Check sheet for the drawn part. Datum: minimum x, y, z corner. Units: mm. A direction names the side the tool comes from. Give positions to 0.01 mm unless a question says otherwise; leave off trailing zeros. Loops run counter-clockwise (first coordinate to the right, second up) from the corner with the lowest first, then second, coordinate; pieces in that order, holes last. Notation, with made-up numbers: (-40, 0.5) -> (7, 0.5) arc R21 ccw to (7, 16.5) -> close; hole circle Ø5 at (69, 83). An arc over 180 degrees is marked (long way). One line per question, with ' | ' between items.
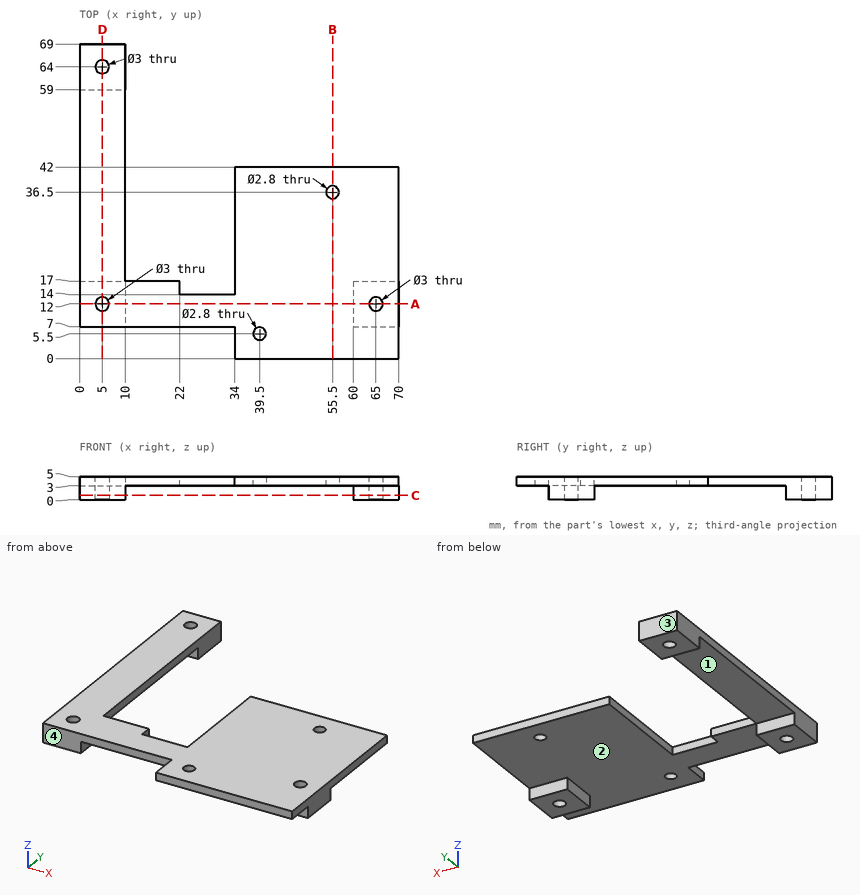
Item 1: Sectioned sample at C-C (z = 0.9). Record the cut outline in (x, y), plus the area to 3 significant figures.
Result:
outline: (0, 7) -> (10, 7) -> (10, 17) -> (0, 17) -> close; (0, 59) -> (10, 59) -> (10, 69) -> (0, 69) -> close; (60, 7) -> (70, 7) -> (70, 17) -> (60, 17) -> close; hole circle Ø3 at (5, 12); hole circle Ø3 at (5, 64); hole circle Ø3 at (65, 12) | area: 279 mm2
Item 2: Sectioned sample at B-B (x = 55.5). Record the cut outline in (y, z), plus the area to 3 significant figures.
Result:
outline: (0, 3) -> (35.1, 3) -> (35.1, 5) -> (0, 5) -> close; (37.9, 3) -> (42, 3) -> (42, 5) -> (37.9, 5) -> close | area: 78.4 mm2
Item 3: Scan lines: probe 1 along X at (y, z) = (13, 3.25); probe 2 along Y at (x, z) = (5, 3.4); probe 3 along X at (y, z) = (64, 3.8). Record each from-to range of solid material in increasing order.
Result:
probe 1: 0 to 3.88, 6.12 to 63.88, 66.12 to 70 | probe 2: 7 to 10.5, 13.5 to 62.5, 65.5 to 69 | probe 3: 0 to 3.5, 6.5 to 10
Item 4: Sectioned sample at D-D (x = 5). Record the cut outline in (y, z), plus the area to 3 significant figures.
Result:
outline: (7, 0) -> (10.5, 0) -> (10.5, 5) -> (7, 5) -> close; (13.5, 0) -> (17, 0) -> (17, 3) -> (59, 3) -> (59, 0) -> (62.5, 0) -> (62.5, 5) -> (13.5, 5) -> close; (65.5, 0) -> (69, 0) -> (69, 5) -> (65.5, 5) -> close | area: 154 mm2
Item 5: Set-up check for the marked faces 3 and 4: record each of +Z, -Z, +X, -X, +Y, -Y from which the full face is reachable in a straight line by a thin tool's end or side.
Result:
face 3: +Z, -Z, +X, -X, +Y | face 4: +Z, -Z, -X, -Y
Item 6: Release check for a two-part mould opening along X. For the marked faces 1 and 2 record: pulls with the +X half, pulls with the -X half, needs draft (parallel to the pull), parting line crosses it, or undercut.
Result:
face 1: needs draft | face 2: undercut
Item 7: Sectioned sample at A-A (y = 12). Record the cut outline in (x, z).
Result:
outline: (0, 0) -> (3.5, 0) -> (3.5, 5) -> (0, 5) -> close; (6.5, 0) -> (10, 0) -> (10, 3) -> (60, 3) -> (60, 0) -> (63.5, 0) -> (63.5, 5) -> (6.5, 5) -> close; (66.5, 0) -> (70, 0) -> (70, 5) -> (66.5, 5) -> close
Item 8: Depth check by flat-ended pin: pin 1 Ø2 at (x, z) = (18, 3.5) entering from +Y; pin 2 Ø4.5 at (x, y) = (55.5, 36.5) entering from -Z; pin 3 Ø1 at (x, z) = (28.5, 4) entering from +Y. Enter the tip coordinate at first touch or a pass-through.
Result:
pin 1: y = 17 | pin 2: z = 3 | pin 3: y = 14
